from build123d import *

# Parameters (mm, degrees)
EXTRUDE_1_DEPTH     = 10
SKETCH_9_W          = 24
SKETCH_9_H          = 40
EXTRUDE_5_DEPTH     = 2
SKETCH_10_R         = 1
EXTRUDE_6_DEPTH     = 24
SKETCH_11_W         = 16
SKETCH_11_H         = 15.152135862
CUT_EXTRUDE_2_DEPTH = 24
SKETCH_12_W         = 2
SKETCH_12_H         = 30
EXTRUDE_7_DEPTH     = 4
SKETCH_13_W         = 5
SKETCH_13_H         = 5
SKETCH_13_W_2       = 4
SKETCH_13_H_2       = 4
SKETCH_15_W         = 2
SKETCH_15_H         = 54
EXTRUDE_8_DEPTH     = 10


with BuildPart() as part:
    # 草图2 → 凸台-拉伸1 (new body)
    with BuildSketch(Plane(origin=(0, 0, 0), x_dir=(1, 0, 0), z_dir=(0, 1, 0))):
        with BuildLine():
            Line((-7, 27), (7, 27))
            ThreePointArc((7, 27), (34, 0), (7, -27))
            Line((7, -27), (-7, -27))
            ThreePointArc((-7, -27), (-34, 0), (-7, 27))
        make_face()
        with BuildLine():
            Line((-7, 25), (7, 25))
            ThreePointArc((7, 25), (32, 0), (7, -25))
            Line((7, -25), (-7, -25))
            ThreePointArc((-7, -25), (-7.50010007, -24.994997498), (-8, -24.979991994))
            Line((-8, -24.979991994), (-8, 24.979991994))
            ThreePointArc((-8, 24.979991994), (-7.50010007, 24.994997498), (-7, 25))
        make_face(mode=Mode.SUBTRACT)
        with BuildLine():
            Line((-12, -24.494897428), (-12, 24.494897428))
            ThreePointArc((-12, 24.494897428), (-32, 0), (-12, -24.494897428))
        make_face(mode=Mode.SUBTRACT)
    extrude(amount=EXTRUDE_1_DEPTH)

    # 草图9 → 凸台-拉伸5 (add)
    with BuildSketch(Plane(origin=(-8, 0, 0), x_dir=(0, 0, -1), z_dir=(1, 0, 0))):
        with Locations((0, 10)):
            Rectangle(SKETCH_9_W, SKETCH_9_H)
    extrude(amount=EXTRUDE_5_DEPTH)

    # 草图10 → 凸台-拉伸6 (add)
    with BuildSketch(Plane(origin=(0, 0, -12), x_dir=(-1, 0, 0), z_dir=(0, 0, -1))):
        with Locations((7, 30)):
            Circle(SKETCH_10_R)
        with Locations((7, -10)):
            Circle(SKETCH_10_R)
    extrude(amount=-EXTRUDE_6_DEPTH)

    # 草图11 → 切除-拉伸2 (cut)
    with BuildSketch(Plane(origin=(-6, 0, 0), x_dir=(0, 0, -1), z_dir=(1, 0, 0))):
        with Locations((0, -7.576067931)):
            Rectangle(SKETCH_11_W, SKETCH_11_H)
    extrude(amount=-CUT_EXTRUDE_2_DEPTH, mode=Mode.SUBTRACT)

    # 草图12 → 凸台-拉伸7 (add)
    with BuildSketch(Plane(origin=(-6, 0, 0), x_dir=(0, 0, -1), z_dir=(1, 0, 0))):
        with Locations((11, 15)):
            Rectangle(SKETCH_12_W, SKETCH_12_H)
        with Locations((-11, 15)):
            Rectangle(SKETCH_12_W, SKETCH_12_H)
    extrude(amount=EXTRUDE_7_DEPTH)

    # 扫描3: sweep along a path in 草图14
    with BuildLine(Plane(origin=(-6, 0, 0), x_dir=(0, 0, -1), z_dir=(1, 0, 0))) as sweep_3_path:
        Line((-2, 7.068163289), (-2, 30))
    # 草图13 → 扫描3 (sweep)
    with BuildSketch(Plane(origin=(0, 30, 0), x_dir=(1, 0, 0), z_dir=(0, 1, 0))):
        with Locations((-4, 0)):
            Rectangle(SKETCH_13_W, SKETCH_13_H)
        with Locations((-4, 0)):
            Rectangle(SKETCH_13_W_2, SKETCH_13_H_2, mode=Mode.SUBTRACT)
    sweep(path=sweep_3_path.line)

    # 草图15 → 凸台-拉伸8 (add)
    with BuildSketch(Plane.XZ):
        with Locations((-33, 0)):
            Rectangle(SKETCH_15_W, SKETCH_15_H)
        with Locations((33, 0)):
            Rectangle(SKETCH_15_W, SKETCH_15_H)
    extrude(amount=-EXTRUDE_8_DEPTH)


solid = part.part
Geometry check sheet. Reference: the model listing, model coordinates, mm. A direction names the side the tool comes from. Round coordinates to 2 decimals unless told otherwise and drop trailing zeros. Loops run counter-clockwise (first coordinate to the right, second up) from the corner with the lowest first, then second, coordinate; pieces in that order, holes last. Notation, with made-up numbers: (9.5, 56.25) -> (47.5, 56.25) arc R20 cw to (47.5, 83.25) -> close; hole circle Ø11 at (46, -35). An arc over 180 degrees is marked (long way). Answer as a JSON object with one key per item and string values. Group by question number.
Item 1: Cross-section at A-A, the plane z = 0. Record the cut outline in (x, y).
Item 2: Release check for a two-part mould opening along X. For faces 6 (the face through (0, 5, 27)), 7 (the face through (34, 5, 0)), 8 (the face through (-1.7, 7.068, 0.2)) record: pulls with the +X half, pulls with the -X half, needs draft (parallel to the pull), parting line crosses it, or undercut.
Item 3: Set-up check for faces 1 (the face through (-32, 5, 18)), 2 (the face through (-4, 19, 2)), 3 (the face through (32, 5, -19)), 4 (the face through (-4, 30, -11)), 5 (the face through (-7, -6, -8)): record each of +Z, -Z, +X, -X, +Y, -Y from which the full face is reachable in a straight line by a thin tool's end or side.
Item 4: Cross-section at D-D, the plane x = -25. Record the cut outline in (y, z), plus the area to 3 significant figures.
Item 5: Cross-section at B-B, the plane y = 27.5. Record the cut outline in (x, z), plus the area to 3 significant figures.
Item 6: Thickness scan on line 1 along Z through (x, y) = (-4.5, 27); line 2 along X through (y, z) = (7, -8); line 3 along Z through (x, y) = (3, 9.5). Record the ranges inside material, lowest first.
Item 7: Cross-section at C-C, the plane z = 13.5. Record the cut outline in (x, y), plus the area to 3 significant figures.
Item 8: Depth check by flat-ended pin: pin 1 Ø4 at (x, z) = (-5.5, 14.5) entering from +Y; pin 2 Ø1 at (x, y) = (-6.5, -8) entering from -Z; pin 3 Ø1.6 at (x, y) = (-7.5, -3.5) entering from +Z; pin 4 Ø1 at (x, z) = (-3, 11) entering from +Y. Enter the tip coordinate at first touch or a pass-through.
Determined:
{
 "1": {"outline": "(-34, 0) -> (-32, 0) -> (-32, 10) -> (-34, 10) -> close; (-12, 0) -> (-6, 0) -> (-6, 30) arc R1 ccw to (-8, 30) -> (-8, 10) -> (-12, 10) -> close; (-2, 7.07) -> (-1.5, 7.07) -> (-1.5, 30) -> (-2, 30) -> close; (32, 0) -> (34, 0) -> (34, 10) -> (32, 10) -> close"},
 "2": {"face 6": "needs draft", "face 7": "pulls with the +X half", "face 8": "undercut"},
 "3": {"face 1": "+Z, +Y, -Y", "face 2": "+Y, -Y", "face 3": "-Z, +Y, -Y", "face 4": "+Z, -Z, +X, +Y", "face 5": "+X, -X, -Y"},
 "4": {"outline": "(0, -20.12) -> (10, -20.12) -> (10, -17.35) -> (0, -17.35) -> close; (0, 17.35) -> (10, 17.35) -> (10, 20.12) -> (0, 20.12) -> close", "area": "55.5 mm²"},
 "5": {"outline": "(-8, -12) -> (-2, -12) -> (-2, -10) -> (-6, -10) -> (-6, -2.5) -> (-1.5, -2.5) -> (-1.5, 2.5) -> (-6, 2.5) -> (-6, 10) -> (-2, 10) -> (-2, 12) -> (-8, 12) -> close; hole (-6, -2) -> (-2, -2) -> (-2, 2) -> (-6, 2) -> close", "area": "70.5 mm²"},
 "6": {"line 1": "z = -12 to -10, -2.5 to -2, 2 to 2.5, 10 to 12", "line 2": "x = -34 to -30.69, -12 to -6, 30.69 to 34", "line 3": "z = -27 to -25, 25 to 27"},
 "7": {"outline": "(-34, 0) -> (-32, 0) -> (-32, 10) -> (-34, 10) -> close; (-30.38, 0) -> (-28.04, 0) -> (-28.04, 10) -> (-30.38, 10) -> close; (-12, 0) -> (-8, 0) -> (-8, 10) -> (-12, 10) -> close; (28.04, 0) -> (30.38, 0) -> (30.38, 10) -> (28.04, 10) -> close; (32, 0) -> (34, 0) -> (34, 10) -> (32, 10) -> close", "area": "127 mm²"},
 "8": {"pin 1": "passes through", "pin 2": "stops at z = -12", "pin 3": "stops at z = 12", "pin 4": "stops at y = 30"}
}
